```python
from build123d import *

# Parameters (mm, degrees)
F1_DEPTH = 25.4
F3_DEPTH = 12.7
F5_DEPTH = 12.7
F6_R     = 6.4018672909
F7_DEPTH = 76.201


with BuildPart() as f1:
    # F0 (on Front) → F1 (new body, symmetric)
    with BuildSketch(Plane.XZ):
        Polygon((0, 38.1), (0, 0), (76.2, 0), (76.2, 12.7), (50.8, 12.7), (50.8, 38.1), (38.1, 38.1), (38.1, 50.8), (12.7, 50.8), align=None)
    extrude(amount=F1_DEPTH, both=True)

    # F2 (on face) → F3 (cut)
    with BuildSketch(Plane.XZ.offset(25.4)):
        Polygon((25.4, 25.4), (50.8, 25.4), (50.8, 38.1), (38.1, 38.1), (38.1, 50.8), (25.4, 50.8), align=None)
    extrude(amount=-F3_DEPTH, mode=Mode.SUBTRACT)

    # F4 (on face) → F5 (cut)
    with BuildSketch(Plane(origin=(0, 25.4, 0), x_dir=(-1, 0, 0), z_dir=(0, 1, 0))):
        Polygon((-50.8, 38.1), (-50.8, 25.4), (-25.4, 25.4), (-25.4, 50.8), (-38.1, 50.8), (-38.1, 38.1), align=None)
    extrude(amount=-F5_DEPTH, mode=Mode.SUBTRACT)

    # F6 (on Right) → F7 (cut, through all)
    with BuildSketch(Plane.YZ):
        with Locations((0, 12.7)):
            Circle(F6_R)
    extrude(amount=F7_DEPTH, mode=Mode.SUBTRACT)


solid = f1.part
```
Build history of the part. All positions in model axes, mm. A direction names the side the tool comes from. Give positions to 0.01 mm unless a question says otherwise; leave off trailing zeros. Loops run counter-clockwise (first coordinate to the right, second up) from the corner with the lowest first, then second, coordinate; pieces in that order, holes last.
Item 1: Slice it at C-C, the plane x = 55.5. List the corners of the cut face in (y, z).
Answers follow:
outline: (-25.4, 0) - (25.4, 0) - (25.4, 12.7) - (6.4, 12.7) arc R6.4 cw to (-6.4, 12.7) - (-25.4, 12.7) - close
Item 2: Slice it at B-B, the plane x = 28. List the corners of the cut face in (y, z).
Answers follow:
outline: (-25.4, 0) - (25.4, 0) - (25.4, 25.4) - (12.7, 25.4) - (12.7, 50.8) - (-12.7, 50.8) - (-12.7, 25.4) - (-25.4, 25.4) - close; hole circle Ø12.8 at (0, 12.7)
Item 3: Slice it at D-D, the plane z = 30. List the corners of the cut face in (x, y), and give its area (3 significant figures).
Answers follow:
outline: (0, -25.4) - (25.4, -25.4) - (25.4, -12.7) - (50.8, -12.7) - (50.8, 12.7) - (25.4, 12.7) - (25.4, 25.4) - (0, 25.4) - close
area: 1,940 mm2
Item 4: Pull direction Y, two halves, no side cores. Call faces 1 (the face through (64, -16, 12.7)), 2 (the face through (35, 12.7, 35)), 3 (the face through (29.1, 2.95, 7.02)): released by +Y, released by -Y, zero draft, split by the parting line, or undercut.
Answers follow:
face 1: zero draft
face 2: released by +Y
face 3: undercut
Item 5: Which spindle directions (+Z, -Z, +X, -X, +Y, -Y) get a long thin tool onto all of the face, cutting with end or side? Do faces 4 (the face through (35, -12.7, 35)), 5 (the face through (25.4, 19, 38)), 6 (the face through (38.1, 0, 44)). Say none if no direction does.
Answers follow:
face 4: +Z, +X, -Y
face 5: +Z, +X, +Y
face 6: +Z, +X, +Y, -Y
Item 6: Drill centre lines: line 1 (Y direction, x = 25, z = 12.7); line 2 (Z direction, x = 25.5, y = -14); line 3 (Z direction, x = 64.5, y = 11). Where is each one in solid material? Low to high.
Answers follow:
line 1: y = -25.4 to -6.4, 6.4 to 25.4
line 2: z = 0 to 25.4
line 3: z = 0 to 12.7
Item 7: Slice it at A-A, the plane y = 0. List the corners of the cut face in (x, z), and give its area (3 significant figures).
Answers follow:
outline: (0, 0) - (76.2, 0) - (76.2, 6.3) - (0, 6.3) - close; (0, 19.1) - (50.8, 19.1) - (50.8, 38.1) - (38.1, 38.1) - (38.1, 50.8) - (12.7, 50.8) - (0, 38.1) - close
area: 1,850 mm2
Item 8: Flat gauge pins, fed straight in: pin 1 (10 mm diameter, centred on x = 44.5, y = -19, fed in from +Z); pin 2 (10 mm diameter, centred on y = -18, z = 35, fed in from +X); pin 3 (20.5 mm diameter, centred on y = 8, z = 20, fed in from +X); pin 4 (10 mm diameter, centred on y = 0, z = 12.7, fed in from +X). Where does each tip first touch, or does it go through?
Answers follow:
pin 1: stops at z = 25.4
pin 2: stops at x = 25.4
pin 3: stops at x = 76.2
pin 4: passes through
